Geometry check sheet. Reference: drawing and pictorial views, mm from the part's lowest x, y, z. A direction names the side the tool comes from. Coordinates: 2 decimals unless noted, no trailing zeros. Write each loop counter-clockwise with the first axis right and the second up, starting at its lowest first coordinate (ties: lowest second). Pieces come first, ordered by that corner, then holes. Notation, with made-up numbers: (-32.5, 26) -> (11.5, 26) arc R18 ccw to (11.5, 58) -> close; hole circle Ø5 at (40.25, 39). An arc over 180 degrees is marked (long way). Answer in a Markdown table with one row per item.
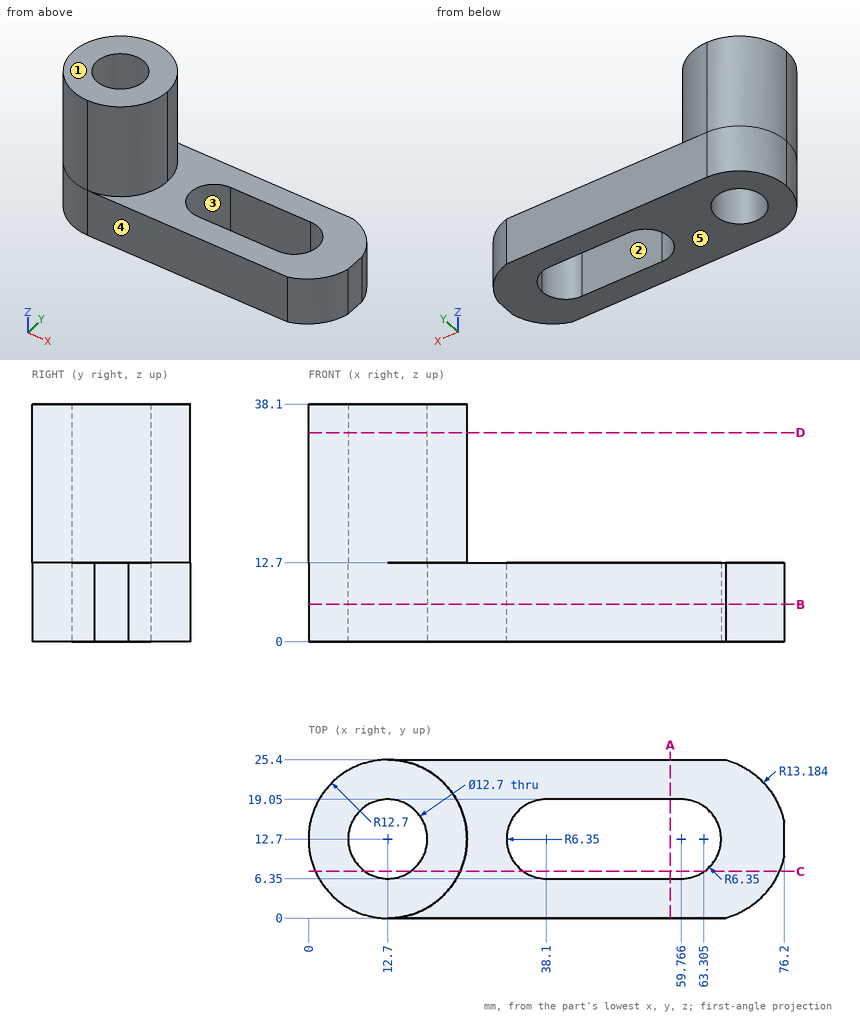
1. Section check A-A, the plane x = 58. Record the boundary of the cut face in (y, z), plus the area to 3 significant figures.
Geometry says:
| item | result |
|---|---|
| outline | (0, 0) -> (6.35, 0) -> (6.35, 12.7) -> (0, 12.7) -> close; (19.05, 0) -> (25.4, 0) -> (25.4, 12.7) -> (19.05, 12.7) -> close |
| area | 161 mm^2 |
2. Mould release check, pull along Y, two halves, no side actions. Record for the marked faces 3, 4 and 5: released by +Y, released by -Y, zero draft, split by the parting line, or undercut.
Geometry says:
| item | result |
|---|---|
| face 3 | undercut |
| face 4 | released by -Y |
| face 5 | zero draft |
3. Section check C-C, the plane y = 7.5. Record the boundary of the cut face in (x, z) (1 decimal), plus the area to 3 significant figures.
Geometry says:
| item | result |
|---|---|
| outline | (1.1, 0) -> (9.1, 0) -> (9.1, 38.1) -> (1.1, 38.1) -> close; (16.3, 0) -> (34.5, 0) -> (34.5, 12.7) -> (24.3, 12.7) -> (24.3, 38.1) -> (16.3, 38.1) -> close; (63.4, 0) -> (75.4, 0) -> (75.4, 12.7) -> (63.4, 12.7) -> close |
| area | 887 mm^2 |
4. Tool access check on the marked faces 1 and 2. Record the directions out of +Z, -Z, +X, -X, +Y, -Y that give a thin tool (end or side, any length) a straight path to the whole face; none if there is none.
Geometry says:
| item | result |
|---|---|
| face 1 | +Z, +X, -X, +Y, -Y |
| face 2 | +Z, -Z |
5. Section check B-B, the plane z = 6. State how many separate pieces and enclosed holes the cut face has, plus the area to 3 significant figures.
Geometry says:
| item | result |
|---|---|
| separate pieces | 1 |
| enclosed holes | 2 |
| area | 1,280 mm^2 |
6. Thickness scan on line 1 (Y direction, x = 45.5, z = 5); line 2 (Z direction, x = 27, y = 20.75); line 3 (X direction, y = 13, z = 28.5). Record the ranges inside material, lowest first. Write a range as from..to.
Geometry says:
| item | result |
|---|---|
| line 1 | 0..6.35, 19.05..25.4 |
| line 2 | 0..12.7 |
| line 3 | 0..6.36, 19.04..25.4 |
7. Section check D-D, the plane z = 33.5. Record the boundary of the cut face in (x, y), plus the area to 3 significant figures.
Geometry says:
| item | result |
|---|---|
| outline | circle Ø25.4 at (12.7, 12.7); hole circle Ø12.7 at (12.7, 12.7) |
| area | 380 mm^2 |
8. Depth check by flat-ended pin: P1, Ø6, axis at x = 30, y = 15.5, coming from the +Z side; P2, Ø4, axis at y = 3, z = 7.5, coming from the -X side; P3, Ø5, axis at y = 22.5, z = 16, coming from the +X side. Enter the tip coordinate at first touch or a pass-through.
Geometry says:
| item | result |
|---|---|
| P1 | z = 12.7 |
| P2 | x = 2.6 |
| P3 | x = 23.09 |
